Source: CAD feature listing. Evaluate the final solid. Frame: model axes, mm. Coordinates: 2 decimals unless noted, no trailing zeros. Put each result on its own line as item: value.
Autodesk Inventor part; units mm, degrees
ref_plane "YZ Plane" through (0, 0, 0) normal (1, 0, 0) x (0, 1, 0)
ref_plane "XZ Plane" through (0, 0, 0) normal (0, 1, 0) x (-1, 0, 0)
ref_plane "XY Plane" through (0, 0, 0) normal (0, 0, 1) x (1, 0, 0)
sketch "Sketch1" plane through (0, 0, 0) normal (0, 1, 0) x (-1, 0, 0)
  ellipse E0 centre (0, 0) end of major axis (14, 0) minor radius 10
  dimension "d0" = 10
  dimension "d1" = 14
ref_plane "Work Plane4" through (0, 38, 0) normal (0, 1, 0) x (1, 0, 0)
sketch "Sketch8" plane through (0, 38, 0) normal (0, 1, 0) x (1, 0, 0)
  circle A0 centre (0, 0) radius 4
  dimension "d13" = 8
loft "Loft2" add profiles "Sketch1", "Sketch8"
fillet "Fillet3" radius 4.29 2 edges at (0, 38, 4) (0, 38, -4)
sketch "Sketch9" plane through (0, 0, 0) normal (1, 0, 0) x (0, 1, 0)
  line L0 (0, 0) -> (34.8018, 0)
  circle A0 centre (7, 0) radius 3
  dimension "d20" = 6
  dimension "d21" = 7
extrude "Extrusion2" cut sketch "Sketch9" along normal through all both and the other way through all
properties part number "landing"
1. Ray query, line 1 along Y through (x, z) = (0.25, 0); line 2 along Z through (x, y) = (-3.5, 7); line 3 along Y through (x, z) = (3.75, -2.5). Return the intervals inside material, ascending.
Numbers:
line 1: y = 0 to 4, 10 to 38
line 2: z = -8.52 to -3, 3 to 8.52
line 3: y = 0 to 5.34, 8.66 to 35.43
2. Pull-direction query (Y, two-part tool) for faces 1 (the cylindrical face through (0, 4, 0)), 2 (the flat face through (0, 0, 0)); classes: pulls with the +Y half, pulls with the -Y half, needs draft (parallel to the pull), parting line crosses it, or undercut.
Numbers:
face 1: undercut
face 2: pulls with the -Y half
3. First-contact query: pin 1 (1.5 mm diameter, centred on y = 23, z = -6, fed in from -X); pin 2 (4 mm diameter, centred on x = 3, y = 21, fed in from +Z); pin 3 (8 mm diameter, centred on y = 11, z = -4, fed in from -X). Flat tips, straight axial feed; report the tip coordinate or a pass-through.
Numbers:
pin 1: stops at x = -4.53
pin 2: stops at z = 6.8
pin 3: stops at x = -11.41
